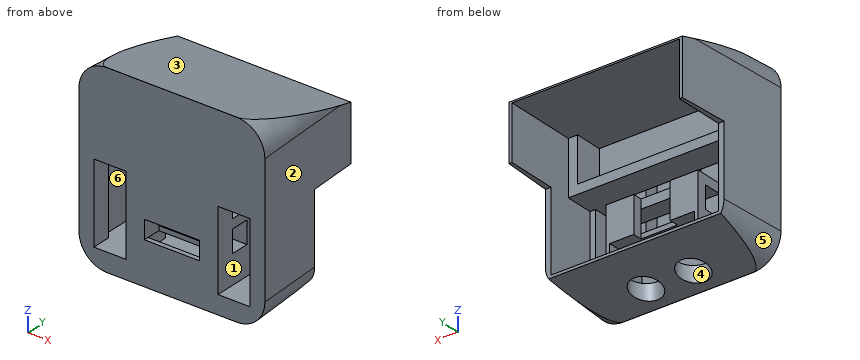
```python
from build123d import *

# Parameters (mm, degrees)
BOSS_EXTRUDE1_DEPTH     = 10
SKETCH2_W               = 17.2
SKETCH2_H               = 43
CUT_EXTRUDE1_DEPTH      = 72.414284285
SKETCH3_W               = 90
SKETCH3_H               = 34
SKETCH3_W_2             = 80
SKETCH3_H_2             = 24
BOSS_EXTRUDE3_DEPTH     = 15
SKETCH4_W               = 49.6
SKETCH4_H               = 5
BOSS_EXTRUDE4_DEPTH     = 10
SKETCH5_W               = 15
SKETCH5_H               = 22
BOSS_EXTRUDE5_DEPTH     = 5
SKETCH6_W               = 90
SKETCH6_H               = 77
BOSS_EXTRUDE6_DEPTH     = 15
BOSS_EXTRUDE8_DEPTH     = 39
CHAMFER1_SIZE           = 64
CHAMFER1_SIZE_2         = 3.354097874
CHAMFER2_SIZE           = 64
CHAMFER2_SIZE_2         = 11.405813635
CHAMFER3_SIZE           = 64
CHAMFER3_SIZE_2         = 13.775745352
CUT_EXTRUDE3_DEPTH      = 95.500525601
CUT_EXTRUDE3_DEPTH_BACK = 95.500525601
SKETCH10_W              = 50
SKETCH10_H              = 27
SKETCH11_W              = 45.5
SKETCH11_H              = 10.5
CUT_EXTRUDE4_DEPTH      = 7.5
SKETCH14_W              = 2.05
SKETCH14_H              = 10.5
BOSS_EXTRUDE9_DEPTH     = 15
SKETCH15_R              = 8
CUT_EXTRUDE5_DEPTH      = 122.227059686
CUT_EXTRUDE6_DEPTH      = 2.5
CUT_EXTRUDE7_REACH      = 97.373
SKETCH18_W              = 29.6
SKETCH18_H              = 45
CUT_EXTRUDE8_DEPTH      = 15
SKETCH21_W              = 29.6
SKETCH21_H              = 35
BOSS_EXTRUDE10_DEPTH    = 2.5


with BuildPart() as part:
    # Sketch1 → Boss-Extrude1 (new body)
    with BuildSketch(Plane(origin=(0, 0, 0), x_dir=(1, 0, 0), z_dir=(0, 1, 0))):
        with BuildLine():
            Line((-35, 50), (35, 50))
            ThreePointArc((35, 50), (45.606601718, 45.606601718), (50, 35))
            Line((50, 35), (50, -35))
            ThreePointArc((50, -35), (45.606601718, -45.606601718), (35, -50))
            Line((35, -50), (-35, -50))
            ThreePointArc((-35, -50), (-45.606601718, -45.606601718), (-50, -35))
            Line((-50, -35), (-50, 35))
            ThreePointArc((-50, 35), (-45.606601718, 45.606601718), (-35, 50))
        make_face()
    extrude(amount=BOSS_EXTRUDE1_DEPTH)

    # Sketch2 → Cut-Extrude1 (cut, through all)
    with BuildSketch(Plane(origin=(0, 10, 0), x_dir=(1, 0, 0), z_dir=(0, 1, 0))):
        with Locations((-33.4, 18.5)):
            Rectangle(SKETCH2_W, SKETCH2_H)
        with Locations((33.4, 18.5)):
            Rectangle(SKETCH2_W, SKETCH2_H)
    extrude(amount=-CUT_EXTRUDE1_DEPTH, mode=Mode.SUBTRACT)

    # Sketch3 → Boss-Extrude3 (add)
    with BuildSketch(Plane(origin=(0, 10, 0), x_dir=(1, 0, 0), z_dir=(0, 1, 0))):
        with Locations((0, -20)):
            Rectangle(SKETCH3_W, SKETCH3_H)
        with Locations((0, -20)):
            Rectangle(SKETCH3_W_2, SKETCH3_H_2, mode=Mode.SUBTRACT)
    extrude(amount=BOSS_EXTRUDE3_DEPTH)

    # Sketch4 → Boss-Extrude4 (add)
    with BuildSketch(Plane(origin=(0, 10, 0), x_dir=(1, 0, 0), z_dir=(0, 1, 0))):
        with Locations((0, 10)):
            Rectangle(SKETCH4_W, SKETCH4_H)
        with Locations((0, 27)):
            Rectangle(SKETCH4_W, SKETCH4_H)
    extrude(amount=BOSS_EXTRUDE4_DEPTH)

    # Sketch5 → Boss-Extrude5 (add)
    with BuildSketch(Plane(origin=(0, 20, 0), x_dir=(1, 0, 0), z_dir=(0, 1, 0))):
        with Locations((-17.3, 18.5)):
            Rectangle(SKETCH5_W, SKETCH5_H)
        with Locations((17.3, 18.5)):
            Rectangle(SKETCH5_W, SKETCH5_H)
    extrude(amount=BOSS_EXTRUDE5_DEPTH)

    # Sketch6 → Boss-Extrude6 (add)
    with BuildSketch(Plane(origin=(0, 10, 0), x_dir=(1, 0, 0), z_dir=(0, 1, 0))):
        with BuildLine():
            Line((-50, 35), (-50, -35))
            ThreePointArc((-50, -35), (-45.606601718, -45.606601718), (-35, -50))
            Line((-35, -50), (35, -50))
            ThreePointArc((35, -50), (45.606601718, -45.606601718), (50, -35))
            Line((50, -35), (50, 35))
            ThreePointArc((50, 35), (45.606601718, 45.606601718), (35, 50))
            Line((35, 50), (-35, 50))
            ThreePointArc((-35, 50), (-45.606601718, 45.606601718), (-50, 35))
        make_face()
        with Locations((0, 1.5)):
            Rectangle(SKETCH6_W, SKETCH6_H, mode=Mode.SUBTRACT)
    extrude(amount=BOSS_EXTRUDE6_DEPTH)

    # Sketch9 → Boss-Extrude8 (add)
    with BuildSketch(Plane(origin=(0, 25, 0), x_dir=(1, 0, 0), z_dir=(0, 1, 0))):
        with BuildLine():
            Line((-50, 35), (-50, -35))
            ThreePointArc((-50, -35), (-45.606601718, -45.606601718), (-35, -50))
            Line((-35, -50), (35, -50))
            ThreePointArc((35, -50), (45.606601718, -45.606601718), (50, -35))
            Line((50, -35), (50, 35))
            ThreePointArc((50, 35), (45.606601718, 45.606601718), (35, 50))
            Line((35, 50), (-35, 50))
            ThreePointArc((-35, 50), (-45.606601718, 45.606601718), (-50, 35))
        make_face()
        with BuildLine():
            Line((-45, 35), (-45, -32))
            Line((-45, -32), (45, -32))
            Line((45, -32), (45, 35))
            ThreePointArc((45, 35), (44.659258263, 37.588190451), (43.660254038, 40))
            Line((43.660254038, 40), (-43.660254038, 40))
            ThreePointArc((-43.660254038, 40), (-44.659258263, 37.588190451), (-45, 35))
        make_face(mode=Mode.SUBTRACT)
    extrude(amount=BOSS_EXTRUDE8_DEPTH)

    # Chamfer1
    # the kernel refuses this chamfer: 64, 3.354097874 mm, written as the material it takes off along each edge
    with BuildSketch(Plane(origin=(-35, 64, 50), x_dir=(0, -0.9999979738662979, 0.002013023422382214), z_dir=(1, 0, 0)), Plane(origin=(50, 64, 35), x_dir=(0.002013023422382214, -0.9999979738662979, 0), z_dir=(0, 0, -1)), Plane(origin=(-50, 64, -35), x_dir=(-0.002013023422382214, -0.9999979738662979, 0), z_dir=(0, 0, 1)), Plane(origin=(35, 64, -50), x_dir=(0, -0.9999979738662979, -0.002013023422382214), z_dir=(-1, 0, 0))) as chamfer1_piece_1:
        Polygon((CHAMFER1_SIZE * 0.999997973866, CHAMFER1_SIZE * 0.00201302342238), (-CHAMFER1_SIZE_2 * 0.00201302342245, CHAMFER1_SIZE_2 * 0.9999979739), (0, 0), align=None)
    extrude(amount=70, mode=Mode.SUBTRACT)
    with BuildSketch(Plane(origin=(35, 64, 35), x_dir=(0, 0, 1), z_dir=(-1, 0, 0))) as chamfer1_piece_2:
        Polygon((15, -CHAMFER1_SIZE), (15 - CHAMFER1_SIZE_2, 0), (15, 0), align=None)
    revolve(axis=Axis((35, 64, 35), (0, 1, 0)), revolution_arc=90, mode=Mode.SUBTRACT)
    with BuildSketch(Plane(origin=(-35, 64, 35), x_dir=(-1, 0, 0), z_dir=(0, 0, -1))) as chamfer1_piece_3:
        Polygon((15, -CHAMFER1_SIZE), (15 - CHAMFER1_SIZE_2, 0), (15, 0), align=None)
    revolve(axis=Axis((-35, 64, 35), (0, 1, 0)), revolution_arc=90, mode=Mode.SUBTRACT)
    with BuildSketch(Plane(origin=(35, 64, -35), x_dir=(1, 0, 0), z_dir=(0, 0, 1))) as chamfer1_piece_4:
        Polygon((15, -CHAMFER1_SIZE), (15 - CHAMFER1_SIZE_2, 0), (15, 0), align=None)
    revolve(axis=Axis((35, 64, -35), (0, 1, 0)), revolution_arc=90, mode=Mode.SUBTRACT)
    with BuildSketch(Plane(origin=(-35, 64, -35), x_dir=(0, 0, -1), z_dir=(1, 0, 0))) as chamfer1_piece_5:
        Polygon((15 - CHAMFER1_SIZE_2, 0), (15, -CHAMFER1_SIZE), (15, 0), align=None)
    revolve(axis=Axis((-35, 64, -35), (0, 1, 0)), revolution_arc=90, mode=Mode.SUBTRACT)

    # Chamfer2
    # the kernel refuses this chamfer: 64, 11.405813635 mm, written as the material it takes off along each edge
    with BuildSketch(Plane(origin=(201.306482971, 64, -46.645902126), x_dir=(0, -0.9982575003065525, -0.05900816114499234), z_dir=(-1, 0, 0))) as chamfer2_piece_1:
        Polygon((CHAMFER2_SIZE * 0.999977671636, CHAMFER2_SIZE * 0.0066825316561), (-CHAMFER2_SIZE_2 * 0.0590081611462, CHAMFER2_SIZE_2 * 0.998257500326), (0, 0), align=None)
    extrude(amount=402.612965942, mode=Mode.SUBTRACT)

    # Chamfer3
    # the kernel refuses this chamfer: 64, 13.775745352 mm, written as the material it takes off along each edge
    with BuildSketch(Plane(origin=(-201.265469314, 64, 46.645902126), x_dir=(0, -0.9981787050157903, 0.06032638604292662), z_dir=(1, 0, 0))) as chamfer3_piece_1:
        Polygon((CHAMFER3_SIZE * 0.999967974892, CHAMFER3_SIZE * 0.00800307379952), (-CHAMFER3_SIZE_2 * 0.060326386045, CHAMFER3_SIZE_2 * 0.99817870505), (0, 0), align=None)
    extrude(amount=402.530938629, mode=Mode.SUBTRACT)

    # Sketch10 → Cut-Extrude3 (cut, two sides: drawn at the far end of the back side and taken through both)
    with BuildSketch(Plane(origin=(0, 1.307501734, 0), x_dir=(0, 0, 1), z_dir=(-1, 0, 0)).offset(-CUT_EXTRUDE3_DEPTH_BACK)):
        with Locations((-22.129843227, 49.192498266)):
            Rectangle(SKETCH10_W, SKETCH10_H)
    extrude(amount=CUT_EXTRUDE3_DEPTH + CUT_EXTRUDE3_DEPTH_BACK, mode=Mode.SUBTRACT)

    # Sketch11 → Cut-Extrude4 (cut)
    with BuildSketch(Plane(origin=(0, 10, 0), x_dir=(1, 0, 0), z_dir=(0, 1, 0))):
        with Locations((0, 34.75)):
            Rectangle(SKETCH11_W, SKETCH11_H)
    extrude(amount=-CUT_EXTRUDE4_DEPTH, mode=Mode.SUBTRACT)

    # Sketch14 → Boss-Extrude9 (add)
    with BuildSketch(Plane(origin=(0, 10, 0), x_dir=(1, 0, 0), z_dir=(0, 1, 0))):
        with Locations((-23.775, 34.75)):
            Rectangle(SKETCH14_W, SKETCH14_H)
        with Locations((23.775, 34.75)):
            Rectangle(SKETCH14_W, SKETCH14_H)
    extrude(amount=BOSS_EXTRUDE9_DEPTH)

    # Sketch15 → Cut-Extrude5 (cut, through all)
    with BuildSketch(Plane.XY.offset(-40)):
        with Locations((-12.75, 12.75)):
            Circle(SKETCH15_R)
        with Locations((12.75, 12.75)):
            Circle(SKETCH15_R)
    extrude(amount=-CUT_EXTRUDE5_DEPTH, mode=Mode.SUBTRACT)

    # Sketch17 → Cut-Extrude6 (cut)
    with BuildSketch(Plane(origin=(0, 0, -29.5), x_dir=(-1, 0, 0), z_dir=(0, 0, -1))):
        Polygon((-9.8, 25), (-22.75, 25), (-22.75, 2.5), (22.75, 2.5), (22.75, 25), (9.8, 25), (9.8, 20), (-9.8, 20), align=None)
    extrude(amount=-CUT_EXTRUDE6_DEPTH, mode=Mode.SUBTRACT)

    # Cut-Extrude7: up to this face of the body (flat: up to its plane)
    cut_extrude7_end = Plane(part.part.faces().sort_by_distance((0, 10, -18.5))[0])
    # Sketch18 → Cut-Extrude7 (cut, up to the picked face)
    with BuildSketch(Plane.XZ, mode=Mode.PRIVATE) as cut_extrude7_sk1:
        with Locations((0, -4.5)):
            Rectangle(SKETCH18_W, SKETCH18_H)
    cut_extrude7_tool1 = split(extrude(cut_extrude7_sk1.sketch, amount=-CUT_EXTRUDE7_REACH, mode=Mode.PRIVATE), bisect_by=cut_extrude7_end, keep=Keep.BOTH, mode=Mode.PRIVATE)
    add(cut_extrude7_tool1.solids().sort_by(Axis((0, 0, -4.5), (0, 1, 0)))[0], mode=Mode.SUBTRACT)

    # Sketch20 → Cut-Extrude8 (cut)
    with BuildSketch(Plane.XZ.offset(-25)):
        with BuildLine():
            Line((-45, -35), (-45, -40))
            Line((-45, -40), (-43.660254038, -40))
            ThreePointArc((-43.660254038, -40), (-44.659258263, -37.588190451), (-45, -35))
        make_face()
        with BuildLine():
            Line((45, -40), (45, -35))
            ThreePointArc((45, -35), (44.659258263, -37.588190451), (43.660254038, -40))
            Line((43.660254038, -40), (45, -40))
        make_face()
    extrude(amount=-CUT_EXTRUDE8_DEPTH, mode=Mode.SUBTRACT)

    # Sketch21 → Boss-Extrude10 (add)
    with BuildSketch(Plane.XZ):
        with Locations((0, 0.5)):
            Rectangle(SKETCH21_W, SKETCH21_H)
    extrude(amount=-BOSS_EXTRUDE10_DEPTH)


solid = part.part
```
Could you check a few things on this model? Use its own coordinates, in mm. Face numbers are marked on the shaded views. A direction names the side the tool comes from. Coordinates: 2 decimals unless noted, no trailing zeros. Write each loop counter-clockwise with the first axis right and the second up, starting at its lowest first coordinate (ties: lowest second). Pieces come first, ordered by that corner, then holes. Notation, with made-up numbers: M 3.5,46.25 L 41.5,46.25 A12 ccw 41.5,57.25 Z; hole C 10.25,64 d11. An arc over 180 degrees is marked long. Answer as CSV lines item,"result". Start each with the question number.
1) I want a section at D-D, the plane z = 27.5. Please give me the cut outline in (x, y), and give its area (3 significant figures).
2) Please list where these lines run through material, in increasing order: line 1 (Y direction, x = -14, z = -15); line 2 (Z direction, x = 16, y = 21); line 3 (Z direction, x = -30.5, y = 22). Write a range as from..to.
3) I want a section at B-B, the plane y = 6. Give the number of separate pieces and of enclosed holes in the cut face, and give its area (3 significant figures).
4) For P1, Ø12, axis at x = 0, z = 22.5, coming from the +Y side; P2, Ø3, axis at y = 6, z = -28.5, coming from the -X side; P3, Ø1.5, axis at y = 12.5, z = -37, coming from the -X side; P4, Ø13, axis at x = -18, z = -20, coming from the -Y side, each with a flat end and sliding along its axis, tell me the tip position at first contact or that it passes through.
5) I want a section at A-A, the plane x = -31. Please give me the cut outline in (y, z).
6) We'd pull the mould along Z, two halves only. Please class the marked faces 1, 2 and 3: +Z half, -Z half, draft (parallel to the pull), parting line (faces both ways), or undercut.
7) For the marked faces 4, 5 and 6, which set-ups out of +Z, -Z, +X, -X, +Y, -Y let a thin tool reach every point of the face, with its end or its side?
Data:
1,outline,"M -50,0 L 50,0 L 46.65,64 L 45,64 L 45,25 L 40,25 L 40,10 L -40,10 L -40,25 L -45,25 L -45,64 L -46.65,64 Z"
1,area,"1,480 mm^2"
2,line 1,"y = 0..2.5, 20..25"
2,line 2,"z = -45.17..-40, -27..-7.5, 3..8, 32..44.39"
2,line 3,"z = -44.94..-40, 3..8, 32..44.12"
3,separate pieces,"2"
3,enclosed holes,"2"
3,area,"5,960 mm^2"
4,P1,"stops at y = 10"
4,P2,"stops at x = -49.76"
4,P3,"stops at x = -49.3"
4,P4,"stops at y = 0"
5,outline,"M 0,-50 L 0.09,-50 L 37,-41.47 L 37,-40 L 0,-40 Z; M 0,3 L 25,3 L 25,8 L 10,8 L 10,32 L 64,32 L 64,32.87 L 0.09,50 L 0,50 Z"
6,face 1,"undercut"
6,face 2,"draft"
6,face 3,"+Z half"
7,face 4,"-Z"
7,face 5,"-Z, -X, +Y"
7,face 6,"+Y"
